For this review, take the finished solid that the model builds, in its own axes (mm). Face numbers are marked on the shaded views. A direction names the side the tool comes from. Coordinates: 2 decimals unless noted, no trailing zeros. Order: outer loops, then holes, each group sorted by start corner. A loop starts at its lowest first (then second) coordinate and runs counter-clockwise, first axis right, second up. Notation, with made-up numbers: (2, 77) -> (17, 77) arc R32 ccw to (17, 116) -> close; hole circle Ø4 at (88.25, 42.5). An arc over 180 degrees is marked (long way). Answer as a JSON object with one key per item and string values. Group by question number.
1) Add section B-B, the plane z = 8.75. Write out the cut boundary in (x, y).
2) Machinability: for the marked faces 5, 6 and 7, which of the approach directions +Z, -Z, +X, -X, +Y, -Y give a long, thin tool a straight path to every point of the face, cutting with its end or side? Answer none if there is none.
3) Draft analysis for pull direction X (two halves, no side actions). For the marked faces 1, 2, 3 and 4, state which applies: +X half, -X half, draft (parallel to the pull), parting line (faces both ways), or undercut.
4) Add section A-A, the plane y = 0. Write out the cut boundary in (x, z).
5) Add section C-C, the plane z = 13. Write out the cut boundary in (x, y).
6) Wall thickness on L1, parallel to Y at x = 17.5, z = 3.5; L2, parallel to Y at x = -11.5, z = 0.85; L3, parallel to Y at x = 35.5, z = 0.8: over which ranges is each line inside the solid? List them lowest first.
7) For pin 1 (4.5 mm diameter, centred on x = 17.5, y = 19.5, fed in from -Z); pin 2 (4 mm diameter, centred on x = -1, z = 11.5, fed in from +Y); pin 3 (2.5 mm diameter, centred on x = 36, y = 7.5, fed in from -Z); pin 4 (4 mm diameter, centred on y = 19, z = 2, fed in from -X), all flat-tipped, find the tip position at first contact; note any pin that passes through.
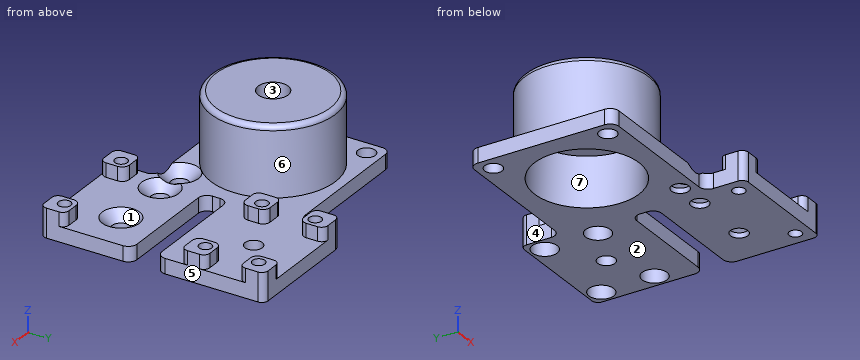
from build123d import *

# Parameters (mm, degrees)
ESQUISSE1_R             = 10.5
ESQUISSE1_R_2           = 1.75
BOSS_EXTRU_1_DEPTH      = 3
ESQUISSE1_3_R           = 12.5
ESQUISSE1_3_R_2         = 3
BOSS_EXTRU_2_DEPTH      = 17
ESQUISSE1_5_R           = 10.5
ENL_V_MAT_EXTRU_1_DEPTH = 10
ESQUISSE4_R             = 1.25
ESQUISSE4_R_2           = 1.75
BOSS_EXTRU_4_DEPTH      = 3
ESQUISSE4_3_W           = 5
ESQUISSE4_3_H           = 5
ESQUISSE4_3_R           = 1.25
BOSS_EXTRU_5_DEPTH      = 5.8
CONG_4_R                = 1.75
CONG_5_R                = 1.25
CONG_6_R                = 1.45
CHANFREIN2_SIZE         = 2
ESQUISSE5_R             = 2.5
ENL_V_MAT_EXTRU_5_DEPTH = 2.8
CONG_7_R                = 1


with BuildPart() as part:
    # Esquisse1 → Boss.-Extru.1 (new body)
    with BuildSketch(Plane.XY):
        with BuildLine():
            Line((0, 14.5), (-14.5, 14.5))
            Line((-14.5, 14.5), (-14.5, -14.5))
            Line((-14.5, -14.5), (14.5, -14.5))
            Line((14.5, -14.5), (14.5, 0))
            ThreePointArc((14.5, 0), (10.253048327, 10.253048327), (0, 14.5))
        make_face()
        Circle(ESQUISSE1_R, mode=Mode.SUBTRACT)
        with Locations((-11.5, 11.5)):
            Circle(ESQUISSE1_R_2, mode=Mode.SUBTRACT)
        with Locations((11.5, -11.5)):
            Circle(ESQUISSE1_R_2, mode=Mode.SUBTRACT)
        with Locations((-11.5, -11.5)):
            Circle(ESQUISSE1_R_2, mode=Mode.SUBTRACT)
    extrude(amount=BOSS_EXTRU_1_DEPTH)

    # Esquisse1<3> → Boss.-Extru.2 (add)
    with BuildSketch(Plane.XY):
        Circle(ESQUISSE1_3_R)
        Circle(ESQUISSE1_3_R_2, mode=Mode.SUBTRACT)
    extrude(amount=BOSS_EXTRU_2_DEPTH)

    # Esquisse1<5> → Enlèv. mat.-Extru.1 (cut)
    with BuildSketch(Plane.XY):
        Circle(ESQUISSE1_5_R)
    extrude(amount=ENL_V_MAT_EXTRU_1_DEPTH, mode=Mode.SUBTRACT)

    # Esquisse4 → Boss.-Extru.4 (add)
    with BuildSketch(Plane(origin=(0, 0, 0), x_dir=(-1, 0, 0), z_dir=(0, 0, -1))):
        with BuildLine():
            Line((-14.5, 22.5), (-38.5, 22.5))
            Line((-38.5, 22.5), (-38.5, 0.85))
            Line((-38.5, 0.85), (-15.5, 0.85))
            Line((-15.5, 0.85), (-15.5, -4.15))
            Line((-15.5, -4.15), (-38.5, -4.15))
            Line((-38.5, -4.15), (-38.5, -22.5))
            Line((-38.5, -22.5), (-14.5, -22.5))
            Line((-14.5, -22.5), (-14.5, 0))
            ThreePointArc((-14.5, 0), (-10.253048327, 10.253048327), (0, 14.5))
            Line((0, 14.5), (-14.5, 14.5))
            Line((-14.5, 14.5), (-14.5, 22.5))
        make_face()
        with Locations((-17.5, 19.5)):
            Circle(ESQUISSE4_R, mode=Mode.SUBTRACT)
        with Locations((-17.750334005, -11.5)):
            Circle(ESQUISSE4_R_2, mode=Mode.SUBTRACT)
        with Locations((-26.5, 12.8)):
            Circle(ESQUISSE4_R_2, mode=Mode.SUBTRACT)
        with Locations((-30.250334005, -11.5)):
            Circle(ESQUISSE4_R_2, mode=Mode.SUBTRACT)
        with Locations((-35.5, 19.5)):
            Circle(ESQUISSE4_R, mode=Mode.SUBTRACT)
        with Locations((-17.5, 8.8)):
            Circle(ESQUISSE4_R, mode=Mode.SUBTRACT)
        with Locations((-17.5, -19.5)):
            Circle(ESQUISSE4_R, mode=Mode.SUBTRACT)
        with Locations((-35.5, 8.8)):
            Circle(ESQUISSE4_R, mode=Mode.SUBTRACT)
        with Locations((-35.5, -19.5)):
            Circle(ESQUISSE4_R, mode=Mode.SUBTRACT)
    extrude(amount=-BOSS_EXTRU_4_DEPTH)

    # Esquisse4<3> → Boss.-Extru.5 (add)
    # profile 1 of 6: a face of its own
    with BuildSketch(Plane(origin=(0, 0, 0), x_dir=(-1, 0, 0), z_dir=(0, 0, -1))):
        with Locations((-17, -20)):
            Rectangle(ESQUISSE4_3_W, ESQUISSE4_3_H)
        with Locations((-17.5, -19.5)):
            Circle(ESQUISSE4_3_R, mode=Mode.SUBTRACT)
    # profile 2 of 6: a face of its own
    with BuildSketch(Plane(origin=(0, 0, 0), x_dir=(-1, 0, 0), z_dir=(0, 0, -1))):
        with Locations((-36, -20)):
            Rectangle(ESQUISSE4_3_W, ESQUISSE4_3_H)
        with Locations((-35.5, -19.5)):
            Circle(ESQUISSE4_3_R, mode=Mode.SUBTRACT)
    # profile 3 of 6: a face of its own
    with BuildSketch(Plane(origin=(0, 0, 0), x_dir=(-1, 0, 0), z_dir=(0, 0, -1))):
        with Locations((-36, 8.3)):
            Rectangle(ESQUISSE4_3_W, ESQUISSE4_3_H)
        with Locations((-35.5, 8.8)):
            Circle(ESQUISSE4_3_R, mode=Mode.SUBTRACT)
    # profile 4 of 6: a face of its own
    with BuildSketch(Plane(origin=(0, 0, 0), x_dir=(-1, 0, 0), z_dir=(0, 0, -1))):
        with Locations((-36, 20)):
            Rectangle(ESQUISSE4_3_W, ESQUISSE4_3_H)
        with Locations((-35.5, 19.5)):
            Circle(ESQUISSE4_3_R, mode=Mode.SUBTRACT)
    # profile 5 of 6: a face of its own
    with BuildSketch(Plane(origin=(0, 0, 0), x_dir=(-1, 0, 0), z_dir=(0, 0, -1))):
        with Locations((-17, 20)):
            Rectangle(ESQUISSE4_3_W, ESQUISSE4_3_H)
        with Locations((-17.5, 19.5)):
            Circle(ESQUISSE4_3_R, mode=Mode.SUBTRACT)
    # profile 6 of 6: a face of its own
    with BuildSketch(Plane(origin=(0, 0, 0), x_dir=(-1, 0, 0), z_dir=(0, 0, -1))):
        with Locations((-17, 8.3)):
            Rectangle(ESQUISSE4_3_W, ESQUISSE4_3_H)
        with Locations((-17.5, 8.8)):
            Circle(ESQUISSE4_3_R, mode=Mode.SUBTRACT)
    extrude(amount=-BOSS_EXTRU_5_DEPTH)

    # Congé4
    cong_4_edges = [part.edges().sort_by_distance(p)[0] for p in [
        (14.5, -14.5, 1.5),
        (-14.5, -14.5, 1.5),
        (-14.5, 14.5, 1.5),
        (38.5, -4.15, 1.5),
        (15.5, -4.15, 1.5),
        (15.5, 0.85, 1.5),
        (38.5, 0.85, 1.5),
        (14.5, 14.5, 1.5),
    ]]
    fillet(cong_4_edges, radius=CONG_4_R)

    # Congé5
    cong_5_edges = [part.edges().sort_by_distance(p)[0] for p in [
        (19.5, -22.5, 4.4),
        (14.5, -17.5, 4.4),
        (38.5, -17.5, 4.4),
        (33.5, -22.5, 4.4),
        (38.5, 10.8, 4.4),
        (38.5, 5.8, 4.4),
        (33.5, 22.5, 4.4),
        (38.5, 17.5, 4.4),
        (19.5, 22.5, 4.4),
        (14.5, 17.5, 4.4),
        (14.5, 10.8, 4.4),
        (14.5, 5.8, 4.4),
        (14.5, -22.5, 2.9),
        (38.5, -22.5, 2.9),
        (38.5, 22.5, 2.9),
        (14.5, 22.5, 2.9),
    ]]
    fillet(cong_5_edges, radius=CONG_5_R)

    # Congé6
    cong_6_edges = [part.edges().sort_by_distance(p)[0] for p in [
        (19.5, -17.5, 4.4),
        (33.5, -17.5, 4.4),
        (33.5, 10.8, 4.4),
        (33.5, 5.8, 4.4),
        (33.5, 17.5, 4.4),
        (19.5, 17.5, 4.4),
        (19.5, 5.8, 4.4),
        (19.5, 10.8, 4.4),
    ]]
    fillet(cong_6_edges, radius=CONG_6_R)

    # Chanfrein2
    # the kernel refuses this chamfer: 2 mm, written as the material it takes off along each edge
    with BuildSketch(Plane(origin=(11.5, -11.5, 3), x_dir=(1, 0, 0), z_dir=(0, -1, 0))) as chanfrein2_piece_1:
        Polygon((1.75 + CHANFREIN2_SIZE, 0), (1.75, -CHANFREIN2_SIZE), (1.75, 0), align=None)
    revolve(axis=Axis((11.5, -11.5, 3), (0, 0, 1)), mode=Mode.SUBTRACT)
    with BuildSketch(Plane(origin=(17.750334005, -11.5, 3), x_dir=(-1, 0, 0), z_dir=(0, -1, 0))) as chanfrein2_piece_2:
        Polygon((1.75 + CHANFREIN2_SIZE, 0), (1.75, CHANFREIN2_SIZE), (1.75, 0), align=None)
    revolve(axis=Axis((17.750334005, -11.5, 3), (0, 0, -1)), mode=Mode.SUBTRACT)
    with BuildSketch(Plane(origin=(30.250334005, -11.5, 3), x_dir=(-1, 0, 0), z_dir=(0, -1, 0))) as chanfrein2_piece_3:
        Polygon((1.75 + CHANFREIN2_SIZE, 0), (1.75, CHANFREIN2_SIZE), (1.75, 0), align=None)
    revolve(axis=Axis((30.250334005, -11.5, 3), (0, 0, -1)), mode=Mode.SUBTRACT)

    # Esquisse5 → Enlèv. mat.-Extru.5 (cut)
    with BuildSketch(Plane(origin=(0, 0, 0), x_dir=(-1, 0, 0), z_dir=(0, 0, -1))):
        with Locations((-35.5, 19.5)):
            Circle(ESQUISSE5_R)
        with Locations((-17.5, 19.5)):
            Circle(ESQUISSE5_R)
        with Locations((-35.5, 8.8)):
            Circle(ESQUISSE5_R)
        with Locations((-17.5, 8.8)):
            Circle(ESQUISSE5_R)
    extrude(amount=-ENL_V_MAT_EXTRU_5_DEPTH, mode=Mode.SUBTRACT)

    # Congé7
    cong_7_edges = [part.edges().sort_by_distance(p)[0] for p in [
        (-12.5, 0, 17),
    ]]
    fillet(cong_7_edges, radius=CONG_7_R)


solid = part.part
Output values:
{
 "1": {"outline": "circle Ø25 at (0, 0); hole circle Ø21 at (0, 0)"},
 "2": {"face 5": "+Z, -Z, +X, +Y, -Y", "face 6": "+Z", "face 7": "-Z"},
 "3": {"face 1": "undercut", "face 2": "draft", "face 3": "undercut", "face 4": "-X half"},
 "4": {"outline": "(-14.5, 0) -> (-10.5, 0) -> (-10.5, 10) -> (-3, 10) -> (-3, 17) -> (-11.5, 17) arc R1 ccw to (-12.5, 16) -> (-12.5, 3) -> (-14.5, 3) -> close; (3, 10) -> (10.5, 10) -> (10.5, 0) -> (15.75, 0) -> (15.75, 3) -> (12.5, 3) -> (12.5, 16) arc R1 ccw to (11.5, 17) -> (3, 17) -> close"},
 "5": {"outline": "circle Ø25 at (0, 0); hole circle Ø6 at (0, 0)"},
 "6": {"L1": "y = -22.5 to -20.75, -18.25 to -17.5, 5.8 to 7.55, 10.05 to 10.8, 17.5 to 18.25, 20.75 to 22.5", "L2": "y = -14.5 to -13.25, -9.75 to 9.75, 13.25 to 14.5", "L3": "y = -22.5 to -20.75, -18.25 to -4.15, 0.85 to 6.3, 11.3 to 17, 22 to 22.5"},
 "7": {"pin 1": "stops at z = 2.8", "pin 2": "stops at y = 12.5", "pin 3": "stops at z = 0", "pin 4": "stops at x = 14.5"}
}
